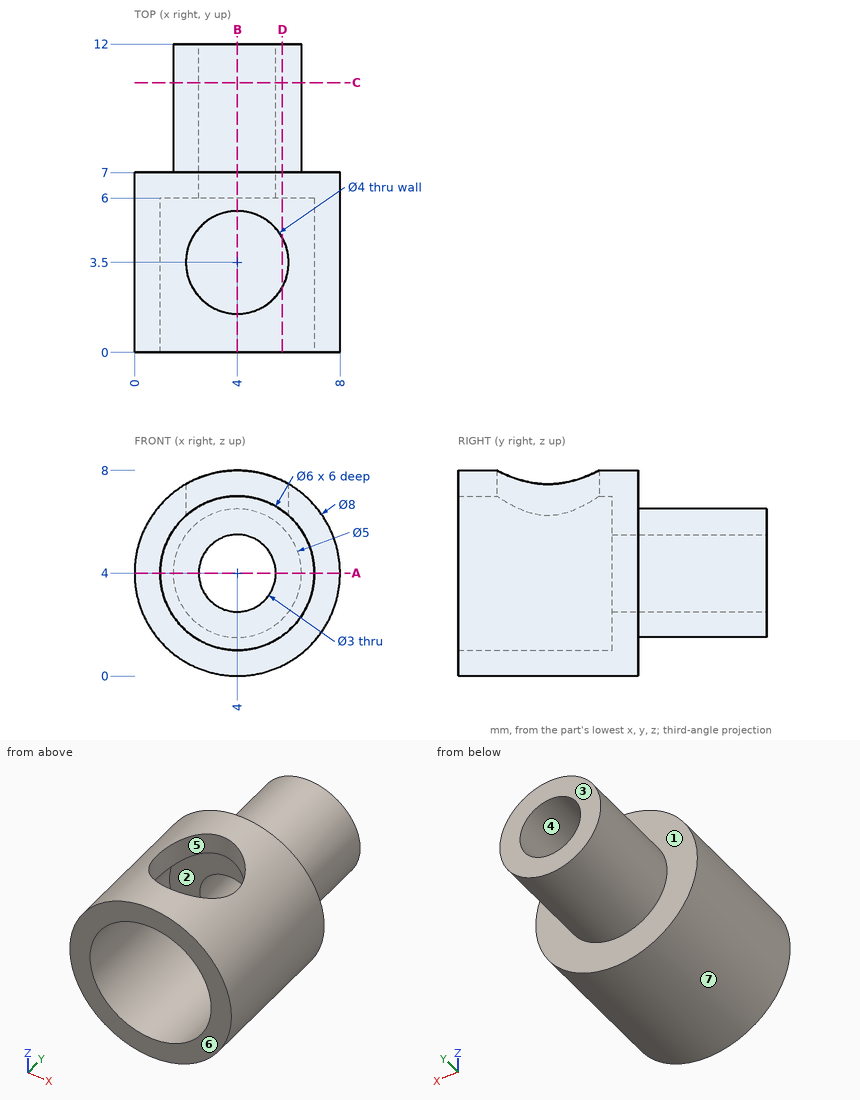
Can you work these out from the drawing? Everything is in mm from the part's minimum corner. A direction names the side the tool comes from. Round coordinates to 2 decimals unless told otherwise and drop trailing zeros. Order: outer loops, then holes, each group sorted by start corner. A loop starts at its lowest first (then second) coordinate and runs counter-clockwise, first axis right, second up.
(1) If we section it at B-B (x = 4): Please give me the cut outline in (y, z).
Results are:
outline: (0, 0) - (7, 0) - (7, 1.5) - (12, 1.5) - (12, 2.5) - (6, 2.5) - (6, 1) - (0, 1) - close; (0, 7) - (1.5, 7) - (1.5, 8) - (0, 8) - close; (5.5, 7) - (6, 7) - (6, 5.5) - (12, 5.5) - (12, 6.5) - (7, 6.5) - (7, 8) - (5.5, 8) - close
(2) On a 3-axis mill with a long thin cutter (end or side, diameter ignored), from which of +Z, -Z, +X, -X, +Y, -Y can I reach the whole of each face in a straight line? I mean the marked faces 1, 2 and 3. Say none if no direction works.
Results are:
face 1: +Y
face 2: -Y
face 3: +Z, -Z, +X, -X, +Y
(3) If we section it at A-A (z = 4): Please give me the cut outline in (x, y).
Results are:
outline: (0, 0) - (1, 0) - (1, 6) - (2.5, 6) - (2.5, 12) - (1.5, 12) - (1.5, 7) - (0, 7) - close; (5.5, 6) - (7, 6) - (7, 0) - (8, 0) - (8, 7) - (6.5, 7) - (6.5, 12) - (5.5, 12) - close
(4) If we section it at D-D (x = 5.75): Please give me the cut outline in (y, z), plus the area to 3 significant figures.
Results are:
outline: (0, 0.4) - (7, 0.4) - (7, 2.21) - (12, 2.21) - (12, 5.79) - (7, 5.79) - (7, 7.6) - (4.47, 7.6) - (4.47, 6.44) - (6, 6.44) - (6, 1.56) - (0, 1.56) - close; (0, 6.44) - (2.53, 6.44) - (2.53, 7.6) - (0, 7.6) - close
area: 36.7 mm2
(5) We'd pull the mould along X, two halves only. Please class the marked faces 4, 5, 6 and 7: +X half, -X half, draft (parallel to the pull), parting line (faces both ways), or undercut.
Results are:
face 4: undercut
face 5: undercut
face 6: draft
face 7: parting line
(6) If I drill on L1, parallel to Z at x = 4, y = 10.75; L2, parallel to Y at x = 4, z = 7.1; L3, parallel to Y at x = 0.5, z = 2.25, over which ranges is the centre line in solid material (lowest first)?
Results are:
L1: z = 1.5 to 2.5, 5.5 to 6.5
L2: y = 0 to 1.5, 5.5 to 7
L3: y = 0 to 7
(7) I'm going to push flat-ended pins straight in: pin 1 (2 mm diameter, centred on x = 3, z = 4.5, fed in from -Y); pin 2 (1.5 mm diameter, centred on y = 10.5, z = 4, fed in from -X). Where does each tip first touch, or does it pass through?
Results are:
pin 1: stops at y = 6
pin 2: stops at x = 1.5
(8) If we section it at C-C (y = 10.5): Please give me the cut outline in (x, z).
Results are:
outline: circle Ø5 at (4, 4); hole circle Ø3 at (4, 4)
